Read the model definition and answer for the solid it produces. Units are mm, in the model's axes. A direction names the side the tool comes from. Give positions to 0.01 mm unless a question says otherwise; leave off trailing zeros. Order: outer loops, then holes, each group sorted by start corner. A loop starts at its lowest first (then second) coordinate and runs counter-clockwise, first axis right, second up. Notation, with made-up numbers: (9, 85.25) - (62, 85.25) arc R19 cw to (62, 102.25) - close; hole circle Ø5 at (84.5, 4). An arc over 180 degrees is marked (long way). Use a Markdown table: item, result. Add a question column.
1. A cutting plane is placed at A-A on x = -26.5. Determine the outline of the cut face in (y, z), and give its area (3 significant figures).
2. For a pull along Z with two mould halves and no side action, classify faces 1 (the flat face through (-43, 3, -127.76)), 2 (the flat face through (-42, 0, -63)), 3 (the flat face through (-43, 5.35, -50)) as released by +Z, released by -Z, zero draft, split by the parting line, or undercut.
3. Consider L1, parallel to Z at x = -6, y = 5.5; L2, parallel to X at y = 6, z = -28.5; L3, parallel to Y at x = -9, z = -75.5. Determine where each line is inside the solid, lowest interval first.
4. A cutting plane is placed at B-B on z = -44.5. Determine the outline of the cut face in (x, y), and give its area (3 significant figures).
5. A flat-ended cylindrical pin translates along its axis: P1, Ø20.5, axis at x = -39, z = -79, coming from the +Y side. Find the tip coordinate at first contact, or state that the pin passes through.
6. Which of the six approach directions +Z, -Z, +X, -X, +Y, -Y give full straight-line access (tool end or side, diameter ignored) to faces 4 (the flat face through (-43, 5.35, -105)), 5 (the flat face through (-33, 6.35, -91))?
Autodesk Inventor part; units mm, degrees
ref_plane "YZ Plane" through (0, 0, 0) normal (1, 0, 0) x (0, 1, 0)
ref_plane "XZ Plane" through (0, 0, 0) normal (0, 1, 0) x (-1, 0, 0)
ref_plane "XY Plane" through (0, 0, 0) normal (0, 0, 1) x (1, 0, 0)
sketch "Sketch1" plane through (0, 0, 0) normal (0, 1, 0) x (-1, 0, 0)
  line L0 (0, 0) -> (85.48, 0)
  line L1 (85.48, 0) -> (85.48, -127.76)
  line L2 (85.48, -127.76) -> (0, -127.76)
  line L3 (0, -127.76) -> (0, 0)
  line L4 (0, 0) -> (7.0711, -7.0711)
  line L5 (0, 0) -> (10, 0) construction
  circle A0 centre (7.0711, -7.0711) radius 4.7625
  dimension "d0" = 85.48
  dimension "d1" = 127.76
  dimension "offsetDiag" = 10
  dimension "d3" = 45
  dimension "d4" = 9.525
extrude "Extrusion1" add sketch "Sketch1" along normal blind 6.35 contours L0 L1 L2 L3 | A0
sketch "Sketch3" plane through (0, 6.35, 0) normal (0, 1, 0) x (1, 0, 0)
  line L0 (0, 0) -> (0, 127.76)
  line L1 (0, 0) -> (-4.3815, 0)
  line L2 (-4.3815, 0) -> (-4.3815, 9.8298)
  line L3 (-4.3815, 9.8298) -> (0, 9.8298)
  line L4 (0, 9.8298) -> (0, 0)
  line L5 (-4.3815, 9.8298) -> (-81.0895, 9.8298)
  line L6 (-81.0895, 9.8298) -> (-81.0895, 35.7298)
  line L7 (-81.0895, 35.7298) -> (-4.3815, 35.7298)
  line L8 (-4.3815, 35.7298) -> (-4.3815, 9.8298)
  line L9 (-81.0895, 35.7298) -> (-82.0895, 35.7298)
  line L10 (-82.0895, 35.7298) -> (-82.0895, 36.7298)
  line L11 (-82.0895, 36.7298) -> (-81.0895, 36.7298)
  line L12 (-81.0895, 36.7298) -> (-81.0895, 35.7298)
  dimension "d23" = 4.3815
  dimension "d24" = 9.8298
  dimension "d25" = 76.708
  dimension "d26" = 25.9
  dimension "d27" = 1
  dimension "d28" = 1
extrude "Extrusion2" cut sketch "Sketch3" against normal blind 1 contours L5 L6 L7 L8
pattern_linear "Rectangular Pattern2" count 4 spacing 27.4 along (0, 0, -1) of "Extrusion2"
properties part number "slide substrate rack"
Output values:
| question | item | result |
|---|---|---|
| 1 | outline | (0, -127.76) - (6.35, -127.76) - (6.35, -117.93) - (5.35, -117.93) - (5.35, -92.03) - (6.35, -92.03) - (6.35, -90.53) - (5.35, -90.53) - (5.35, -64.63) - (6.35, -64.63) - (6.35, -63.13) - (5.35, -63.13) - (5.35, -37.23) - (6.35, -37.23) - (6.35, -35.73) - (5.35, -35.73) - (5.35, -9.83) - (6.35, -9.83) - (6.35, 0) - (0, 0) - close |
| 1 | area | 708 mm² |
| 2 | face 1 | released by -Z |
| 2 | face 2 | zero draft |
| 2 | face 3 | undercut |
| 3 | L1 | -127.76 to -117.93, -92.03 to -90.53, -64.63 to -63.13, -37.23 to -35.73, -9.83 to 0 |
| 3 | L2 | -85.48 to -81.09, -4.38 to 0 |
| 3 | L3 | 0 to 5.35 |
| 4 | outline | (-85.48, 0) - (0, 0) - (0, 6.35) - (-4.38, 6.35) - (-4.38, 5.35) - (-81.09, 5.35) - (-81.09, 6.35) - (-85.48, 6.35) - close |
| 4 | area | 466 mm² |
| 5 | P1 | y = 5.35 |
| 6 | face 4 | +Y |
| 6 | face 5 | +Z, -Z, +X, -X, +Y |
